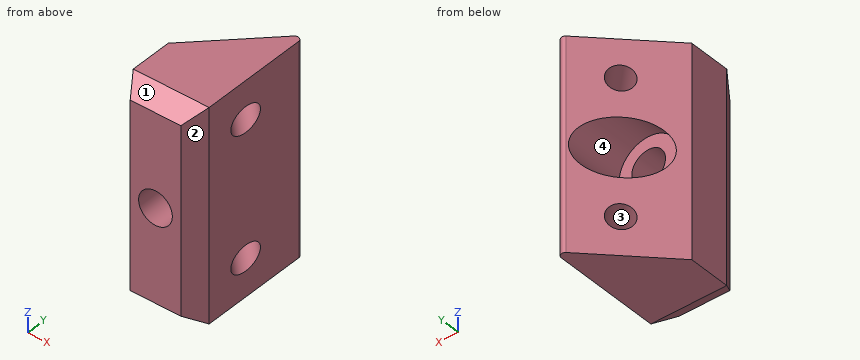
```python
from build123d import *

# Parameters (mm, degrees)
F1_DEPTH = 25
F2_SIZE2 = 2.25
F2_SIZE  = 1.5
F4_D     = 4
F6_D     = 3
F9_D     = 7
F9_DEPTH = 7.5438932188


# Not quite as in the source:
# - a feature names something its author has since deleted; it is built from what else it names


with BuildPart() as f1:
    # F0 (on Top) → F1 (new body)
    with BuildSketch(Plane.XY):
        with BuildLine():
            Line((2.7078659423, 3.7500000373), (2.7078659423, 8.7500000373))
            Line((2.7078659423, 8.7500000373), (2.7078659423, 16.5428932561))
            ThreePointArc((2.7078659423, 16.5428932561), (2.3992076585, 17.0048330223), (1.8543125517, 16.8964466467))
            Line((1.8543125517, 16.8964466467), (-6.2921340577, 8.7500000373))
            Line((-6.2921340577, 8.7500000373), (-6.2921340577, 3.7500000373))
            Line((-6.2921340577, 3.7500000373), (-4.7921340577, 1.5000000373))
            Line((-4.7921340577, 1.5000000373), (1.2078659423, 1.5000000373))
            Line((1.2078659423, 1.5000000373), (2.7078659423, 3.7500000373))
        make_face()
    extrude(amount=F1_DEPTH)

    # F2
    f2_edges = [f1.edges().sort_by_distance(p)[0] for p in [
        (-1.792134, 1.5, 25),
        (-1.792134, 1.5, 0),
    ]]
    chamfer(f2_edges, length=F2_SIZE, length2=F2_SIZE2)

    # F4 (through all)
    with Locations(Plane.XZ.offset(-1.5000000373)):
        with Locations((-1.7921340577, 12.5)):
            Hole(F4_D / 2)

    # F6 (through all)
    with Locations(Plane(origin=(-7.5210670475, 7.5210670475, 0), x_dir=(-0.7071067812, -0.7071067812, 0), z_dir=(-0.7071067812, 0.7071067812, 0))):
        with Locations((-8.2587889815, 4.5), (-8.2587889815, 20.5)):
            Hole(F6_D / 2)

    # F9 (through all, one way)
    with BuildSketch(Plane.XZ.offset(-9.5000000373)):
        with Locations((-1.7921340577, 12.5)):
            Circle(F9_D / 2)
    extrude(amount=-F9_DEPTH, mode=Mode.SUBTRACT)


solid = f1.part
```
The listing builds one solid part. Answer for the finished solid, in the listing's coordinates (mm). Face numbers are marked on the shaded views. Coordinates: 2 decimals unless noted, no trailing zeros. Order: outer loops, then holes, each group sorted by start corner. A loop starts at its lowest first (then second) coordinate and runs counter-clockwise, first axis right, second up. Notation, with made-up numbers: M 2.5,48 L 51.5,48 A21 ccw 51.5,75 Z; hole C -27.75,29.25 d4. An arc over 180 degrees is marked long. Answer as a JSON object with one key per item and string values. Group by question number.
1. Straight lines are drawn through the part: line 1 (Z direction, x = 0, y = 11); line 2 (X direction, y = 9.75, z = 7.75); line 3 (Z direction, x = -0.5, y = 6.75). For each, find the intervals that lie inside material, in ascending order.
2. Section D-D on x = -0.25 is taken. State how many separate pieces and enclosed holes the cut face has, then the cut area to 3 significant figures.
3. Section A-A on z = 12.5 is taken. Write down the section's boundary in (x, y), then the cut area to 3 significant figures.
4. Section B-B on y = 4.75 is taken. Write down the section's boundary in (x, z).
5. Flat-ended cylindrical pins translate along their axes: P1, Ø1.5, axis at y = 13.5, z = 8, coming from the -X side; P2, Ø2, axis at x = 0, z = 13, coming from the +Y side; P3, Ø3, axis at x = -1.79, z = 12.5, coming from the +Y side. Find the tip coordinate at first contact, or state that the pin passes through.
6. Section C-C on z = 23 is taken. Write down the section's boundary in (x, y), then the cut area to 3 significant figures.
7. Determine the mould class of the marked faces 1, 2, 3 and 4 for opening direction Z: released by +Z, released by -Z, zero draft, split by the parting line, or undercut.
Values follow:
{
 "1": {"line 1": "0 to 3.08, 5.92 to 9.49, 15.51 to 19.08, 21.92 to 25", "line 2": "-5.29 to 2.71", "line 3": "0 to 10.97, 14.03 to 25"},
 "2": {"separate pieces": "2", "enclosed holes": "2", "area": "255 mm2"},
 "3": {"outline": "M -6.29,3.75 L -4.79,1.5 L -3.79,1.5 L -3.79,9.5 L -5.29,9.5 L -5.29,9.75 L -6.29,8.75 Z; M 0.21,1.5 L 1.21,1.5 L 2.71,3.75 L 2.71,16.54 A0.5 ccw 1.85,16.9 L 1.71,16.75 L 1.71,9.5 L 0.21,9.5 Z", "area": "43.8 mm2"},
 "4": {"outline": "M -6.29,0 L 2.71,0 L 2.71,25 L -6.29,25 Z; hole C -1.79,12.5 d4"},
 "5": {"P1": "x = -2.29", "P2": "y = 9.5", "P3": "through"},
 "6": {"outline": "M -6.29,3.75 L -4.79,1.5 L 1.21,1.5 L 2.71,3.75 L 2.71,16.54 A0.5 ccw 1.85,16.9 L -6.29,8.75 Z", "area": "102 mm2"},
 "7": {"face 1": "released by +Z", "face 2": "zero draft", "face 3": "undercut", "face 4": "undercut"}
}
